```python
from build123d import *

# Parameters (mm, degrees)
SKETCH1_W           = 220
SKETCH1_H           = 220
BOSS_EXTRUDE1_DEPTH = 30
SKETCH2_R           = 61.5
SKETCH2_R_2         = 50.5
CUT_EXTRUDE1_DEPTH  = 6
SKETCH3_R           = 50.5
SKETCH3_R_2         = 40
CUT_EXTRUDE2_DEPTH  = 4.5
SKETCH4_R           = 40
CUT_EXTRUDE3_DEPTH  = 3.5
SKETCH5_R           = 40
SKETCH6_R           = 20
SKETCH8_R           = 20
CUT_EXTRUDE4_DEPTH  = 1
CHAMFER1_SIZE       = 1.5
CHAMFER1_SIZE_2     = 1.399267753


with BuildPart() as part:
    # Sketch1 → Boss-Extrude1 (new body)
    with BuildSketch(Plane(origin=(0, 0, 0), x_dir=(1, 0, 0), z_dir=(0, 1, 0))):
        Rectangle(SKETCH1_W, SKETCH1_H)
    extrude(amount=BOSS_EXTRUDE1_DEPTH)

    # Sketch2 → Cut-Extrude1 (cut)
    with BuildSketch(Plane(origin=(0, 30, 0), x_dir=(1, 0, 0), z_dir=(0, 1, 0))):
        with Locations(Location((0, 0, 0), (0, 0, 270))):
            Circle(SKETCH2_R)
        with Locations(Location((0, 0, 0), (0, 0, 270))):
            Circle(SKETCH2_R_2, mode=Mode.SUBTRACT)
    extrude(amount=-CUT_EXTRUDE1_DEPTH, mode=Mode.SUBTRACT)

    # Sketch3 → Cut-Extrude2 (cut)
    with BuildSketch(Plane(origin=(0, 30, 0), x_dir=(1, 0, 0), z_dir=(0, 1, 0))):
        with Locations(Location((0, 0, 0), (0, 0, 270))):
            Circle(SKETCH3_R)
        with Locations(Location((0, 0, 0), (0, 0, 270))):
            Circle(SKETCH3_R_2, mode=Mode.SUBTRACT)
    extrude(amount=-CUT_EXTRUDE2_DEPTH, mode=Mode.SUBTRACT)

    # Sketch4 → Cut-Extrude3 (cut)
    with BuildSketch(Plane(origin=(0, 30, 0), x_dir=(1, 0, 0), z_dir=(0, 1, 0))):
        with Locations(Location((0, 0, 0), (0, 0, 270))):
            Circle(SKETCH4_R)
    extrude(amount=-CUT_EXTRUDE3_DEPTH, mode=Mode.SUBTRACT)

    # Sketch5 → Loft1 section 0
    with BuildSketch(Plane(origin=(0, 26.5, 0), x_dir=(1, 0, 0), z_dir=(0, 1, 0))):
        Circle(SKETCH5_R)
    # Sketch6 → Loft1 section 1
    with BuildSketch(Plane(origin=(0, 28, 0), x_dir=(1, 0, 0), z_dir=(0, 1, 0))):
        Circle(SKETCH6_R)
    loft()

    # Sketch8 → Cut-Extrude4 (cut)
    with BuildSketch(Plane(origin=(0, 28, 0), x_dir=(1, 0, 0), z_dir=(0, 1, 0))):
        with Locations(Location((0, 0, 0), (0, 0, 270))):
            Circle(SKETCH8_R)
    extrude(amount=-CUT_EXTRUDE4_DEPTH, mode=Mode.SUBTRACT)

    # Chamfer1
    # the kernel refuses this chamfer: 1.5, 1.399267753 mm, written as the material it takes off along each edge
    with BuildSketch(Plane(origin=(0, 28, 0), x_dir=(1, 0, 0), z_dir=(0, 0, 1))) as chamfer1_piece_1_section:
        Polygon((20 + CHAMFER1_SIZE * 0.997199309888, -CHAMFER1_SIZE * 0.0747899482416), (20, -CHAMFER1_SIZE_2), (20, 0), align=None)
    chamfer1_piece_1 = revolve(axis=Axis((0, 28, 0), (0, 1, 0)), revolution_arc=270, mode=Mode.PRIVATE)
    chamfer1_piece_1 = split(chamfer1_piece_1, bisect_by=Plane(origin=(-14.829664254, 27, -14.829664254), z_dir=(0, 1, 0)), keep=Keep.TOP, mode=Mode.PRIVATE)
    add(chamfer1_piece_1, mode=Mode.SUBTRACT)
    with BuildSketch(Plane(origin=(0, 28, 0), x_dir=(0, 0, 1), z_dir=(-1, 0, 0))) as chamfer1_piece_2_section:
        Polygon((20 + CHAMFER1_SIZE * 0.997199309888, -CHAMFER1_SIZE * 0.0747899482416), (20, -CHAMFER1_SIZE_2), (20, 0), align=None)
    chamfer1_piece_2 = revolve(axis=Axis((0, 28, 0), (0, 1, 0)), revolution_arc=90, mode=Mode.PRIVATE)
    chamfer1_piece_2 = split(chamfer1_piece_2, bisect_by=Plane(origin=(14.836241564, 27, 14.836241564), z_dir=(0, 1, 0)), keep=Keep.TOP, mode=Mode.PRIVATE)
    add(chamfer1_piece_2, mode=Mode.SUBTRACT)


solid = part.part
```
Source: CAD feature listing. Evaluate the final solid. Frame: model axes, mm. A direction names the side the tool comes from. Give positions to 0.01 mm unless a question says otherwise; leave off trailing zeros. Order: outer loops, then holes, each group sorted by start corner. A loop starts at its lowest first (then second) coordinate and runs counter-clockwise, first axis right, second up.
(1) Pull-direction query (X, two-part tool) for faces 1 (the face through (-2, 0, -2)), 2 (the face through (0, 27, 0)), 3 (the face through (-110, 15, 2)); classes: +X half, -X half, draft (parallel to the pull), parting line (faces both ways), or undercut.
(2) Material intervals for line 1 along X through (y, z) = (26.3, 0); line 2 along Y through (x, z) = (-1, 14.5); line 3 along Y through (x, z) = (-15.5, 57), sorted ascending.
(3) Contact query for flat-ended pins moving along their axis: P1, Ø5, axis at x = -11, z = 42, coming from the +Y side; P2, Ø8, axis at x = 11.5, z = 29.5, coming from the +Y side; P3, Ø12.5, axis at x = -10, z = -1.5, coming from the +Y side. Output: stop coordinate, or through.
(4) Access query for faces 4 (the face through (-39.05, 26.01, -8.67)), 5 (the face through (-2, 15, -110)). Directions: +Z, -Z, +X, -X, +Y, -Y. A direction counts if a zero-diameter tool reaches every point of the face in a straight line with its end or side. Return the directions, or none.
(5) Section query A-A (x = 0). Return the cut outline in (y, z).
Outcome:
1. face 1: draft
1. face 2: undercut
1. face 3: -X half
2. line 1: x = -110 to -61.5, -40 to 40, 61.5 to 110
2. line 2: y = 0 to 27
2. line 3: y = 0 to 24
3. P1: stops at y = 25.5
3. P2: stops at y = 27.43
3. P3: stops at y = 27
4. face 4: +Y
4. face 5: -Z, +X, -X, +Y, -Y
5. outline: (0, -110) - (30, -110) - (30, -61.5) - (24, -61.5) - (24, -50.5) - (25.5, -50.5) - (25.5, -40) - (26.5, -40) - (27.89, -21.5) - (27, -20.46) - (27, 20.46) - (27.89, 21.5) - (26.5, 40) - (25.5, 40) - (25.5, 50.5) - (24, 50.5) - (24, 61.5) - (30, 61.5) - (30, 110) - (0, 110) - close
